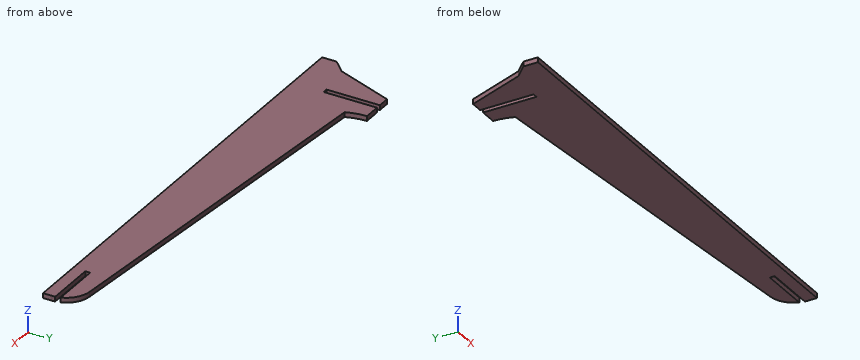
from build123d import *

# Parameters (mm, degrees)
RESSALTO_EXTRUS_O1_DEPTH = 2


with BuildPart() as part:
    # Esboço1 → Ressalto-extrusão1 (new body)
    with BuildSketch(Plane.XY):
        with BuildLine():
            Line((-99.38960786, -14.180843063), (-99.38960786, -8.180843063))
            Line((-99.38960786, -8.180843063), (-94.38960786, -3.180843063))
            Line((-94.38960786, -3.180843063), (-85.410682211, 20.819156937))
            Line((-85.410682211, 20.819156937), (-80.410682211, 20.819156937))
            Line((-80.410682211, 20.819156937), (-80.410682211, -1.180843063))
            Line((-80.410682211, -1.180843063), (-78.410682211, -1.180843063))
            Line((-78.410682211, -1.180843063), (-78.410682211, 20.819156937))
            Line((-78.410682211, 20.819156937), (-71.410682211, 20.819156937))
            ThreePointArc((-71.410682211, 20.819156937), (-71.004691587, 16.614538042), (-69.801720857, 12.565277632))
            Line((-69.801720857, 12.565277632), (86.438560019, -0.41864307))
            ThreePointArc((86.438560019, -0.41864307), (91.771593682, -2.507769172), (95.083402302, -7.180843063))
            Line((95.083402302, -7.180843063), (74.537713689, -7.180843063))
            Line((74.537713689, -7.180843063), (74.537713689, -9.180843063))
            Line((74.537713689, -9.180843063), (95.537713689, -9.180843063))
            ThreePointArc((95.537713689, -9.180843063), (95.59220599, -9.781470716), (95.61039214, -10.384290965))
            Line((95.61039214, -10.384290965), (95.61039214, -14.180843063))
            Line((95.61039214, -14.180843063), (-99.38960786, -14.180843063))
        make_face()
    extrude(amount=RESSALTO_EXTRUS_O1_DEPTH)


solid = part.part
The model under review builds one solid part; all positions refer to its coordinate system, in mm. Round coordinates to 2 decimals unless told otherwise and drop trailing zeros. Write each loop counter-clockwise with the first axis right and the second up, starting at its lowest first coordinate (ties: lowest second). Pieces come first, ordered by that corner, then holes. Notation, with made-up numbers: (3, 8) - (38, 8) arc R28 ccw to (38, 46) - close; hole circle Ø2 at (-10, 78). An arc over 180 degrees is marked (long way). One line per item, written item: value. Start each with the question number.
1. To check wall thickness, follow L1, parallel to X at y = 16.5, z = 0.45; L2, parallel to Y at x = -2.5, z = 1.5; L3, parallel to Y at x = -52, z = 1.35. State the ranges of each line that lie inside material, in increasing order. Write a range as from..to.
2. Clearance check with flat-ended pins moving along their axes: P1, Ø4, axis at x = -51.5, y = 13, coming from the +Z side; P2, Ø0.6, axis at x = 83.5, z = 1, coming from the +Y side; P3, Ø6, axis at x = -27, y = 15, coming from the +Z side; P4, Ø1, axis at y = -8.5, z = 1.5, coming from the +X side. State where each tip first meets the part, or that it passes through.
3. Consider section C-C on z = 0.7. Write out the cut boundary in (x, y).
4. Consider section A-A on x = 82.5. Write out the cut boundary in (y, z), and give its area (3 significant figures).
5. Consider section B-B on y = 18. Write out the cut boundary in (x, z), and give its area (3 significant figures).
6. Consider section D-D on x = 55.5. Write out the cut boundary in (y, z).
Checks:
1. L1: x = -87.03..-80.41, -78.41..-70.98
1. L2: y = -14.18..6.97
1. L3: y = -14.18..11.09
2. P1: stops at z = 2
2. P2: stops at y = -0.15
2. P3: passes through
2. P4: stops at x = 74.54
3. outline: (-99.39, -14.18) - (95.61, -14.18) - (95.61, -10.38) arc R10 ccw to (95.54, -9.18) - (74.54, -9.18) - (74.54, -7.18) - (95.08, -7.18) arc R10 ccw to (86.44, -0.42) - (-69.8, 12.57) arc R21.98 cw to (-71.41, 20.82) - (-78.41, 20.82) - (-78.41, -1.18) - (-80.41, -1.18) - (-80.41, 20.82) - (-85.41, 20.82) - (-94.39, -3.18) - (-99.39, -8.18) - close
4. outline: (-14.18, 0) - (-9.18, 0) - (-9.18, 2) - (-14.18, 2) - close; (-7.18, 0) - (-0.09, 0) - (-0.09, 2) - (-7.18, 2) - close
4. area: 24.2 mm^2
5. outline: (-86.47, 0) - (-80.41, 0) - (-80.41, 2) - (-86.47, 2) - close; (-78.41, 0) - (-71.23, 0) - (-71.23, 2) - (-78.41, 2) - close
5. area: 26.5 mm^2
6. outline: (-14.18, 0) - (2.15, 0) - (2.15, 2) - (-14.18, 2) - close
